from build123d import *

# Parameters (mm, degrees)
CYLINDER_R        = 0.4
CYLINDER_DEPTH    = 4.6
CYLINDER001_R     = 0.4
CYLINDER001_DEPTH = 4.6
CYLINDER002_R     = 0.4
CYLINDER002_DEPTH = 4.6
CYLINDER003_R     = 0.4
CYLINDER003_DEPTH = 4.6
BOX003_W          = 12.8
BOX003_H          = 16.299999
BOX003_DEPTH      = 2
BOX002_W          = 3.4
BOX002_H          = 18.299999
BOX002_DEPTH      = 2
BOX001_W          = 3.4
BOX001_H          = 18.299999
BOX001_DEPTH      = 2
BOX_W             = 12.8
BOX_H             = 18.299999
BOX_DEPTH         = 20.299999
CHAMFER_SIZE      = 3
FILLET_R          = 0.6


with BuildPart() as pin4:
    # Cylinder → Cylinder (new body)
    with BuildSketch(Plane(origin=(1.4, 1.65, -2.6), x_dir=(1, 0, 0), z_dir=(0, 0, 1))):
        Circle(CYLINDER_R)
    extrude(amount=CYLINDER_DEPTH)


with BuildPart() as pin3:
    # Cylinder001 → Cylinder001 (new body)
    with BuildSketch(Plane(origin=(11.4, 1.65, -2.6), x_dir=(1, 0, 0), z_dir=(0, 0, 1))):
        Circle(CYLINDER001_R)
    extrude(amount=CYLINDER001_DEPTH)


with BuildPart() as pin2:
    # Cylinder002 → Cylinder002 (new body)
    with BuildSketch(Plane(origin=(11.4, 16.65, -2.6), x_dir=(1, 0, 0), z_dir=(0, 0, 1))):
        Circle(CYLINDER002_R)
    extrude(amount=CYLINDER002_DEPTH)


with BuildPart() as pin1:
    # Cylinder003 → Cylinder003 (new body)
    with BuildSketch(Plane(origin=(1.4, 16.65, -2.6), x_dir=(1, 0, 0), z_dir=(0, 0, 1))):
        Circle(CYLINDER003_R)
    extrude(amount=CYLINDER003_DEPTH)


with BuildPart() as box003:
    # Box003 → Box003 (new body)
    with BuildSketch(Plane(origin=(0, 1, 0), x_dir=(1, 0, 0), z_dir=(0, 0, 1))):
        with Locations((6.4, 8.149999)):
            Rectangle(BOX003_W, BOX003_H)
    extrude(amount=BOX003_DEPTH)


with BuildPart() as right_cutout:
    # Box002 → Box002 (new body)
    with BuildSketch(Plane(origin=(9.4, 0, 0), x_dir=(1, 0, 0), z_dir=(0, 0, 1))):
        with Locations((1.7, 9.149999)):
            Rectangle(BOX002_W, BOX002_H)
    extrude(amount=BOX002_DEPTH)


with BuildPart() as left_cutout:
    # Box001 → Box001 (new body)
    with BuildSketch(Plane.XY):
        with Locations((1.7, 9.149999)):
            Rectangle(BOX001_W, BOX001_H)
    extrude(amount=BOX001_DEPTH)


with BuildPart() as obj1:
    # Box → Box (new body)
    with BuildSketch(Plane.XY):
        with Locations((6.4, 9.149999)):
            Rectangle(BOX_W, BOX_H)
    extrude(amount=BOX_DEPTH)

    # Cut: cut left_cutout
    add(left_cutout.part, mode=Mode.SUBTRACT)

    # Cut001: cut right_cutout
    add(right_cutout.part, mode=Mode.SUBTRACT)

    # Cut002: cut Box003
    add(box003.part, mode=Mode.SUBTRACT)

    # Chamfer
    chamfer_edges = [obj1.edges().sort_by_distance(p)[0] for p in [
        (6.4, 18.299999, 20.299999),
    ]]
    chamfer(chamfer_edges, length=CHAMFER_SIZE)

    # Fillet
    fillet_edges = [obj1.edges().sort_by_distance(p)[0] for p in [
        (0, 7.65, 20.299999),
        (6.4, 0, 20.299999),
        (12.8, 7.65, 20.299999),
        (0, 0, 11.15),
        (0, 18.299999, 9.65),
        (12.8, 0, 11.15),
        (12.8, 18.299999, 9.65),
    ]]
    fillet(fillet_edges, radius=FILLET_R)

    # Fusion: union Pin4, Pin3, Pin2, Pin1
    add(pin4.part)
    add(pin3.part)
    add(pin2.part)
    add(pin1.part)


solid = obj1.part
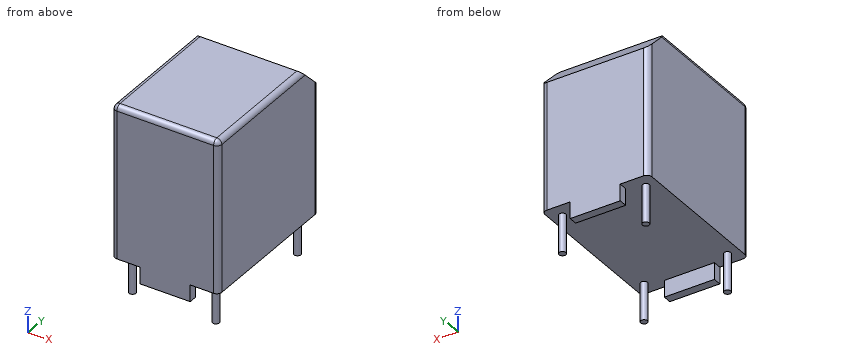
Work out the finished part from the listing and answer in its coordinate system (mm). Give positions to 0.01 mm unless a question says otherwise; leave off trailing zeros. Loops run counter-clockwise (first coordinate to the right, second up) from the corner with the lowest first, then second, coordinate; pieces in that order, holes last. Notation, with made-up numbers: (78.5, -26.75) -> (131.5, -26.75) arc R10 cw to (131.5, -17.75) -> close; hole circle Ø8 at (60.25, 5). An arc over 180 degrees is marked (long way). Use a Markdown table: item, result. Add a question column.
1. Find the intervals of material crossed by probe 1 along Z at (x, y) = (3.5, 14.5); probe 2 along Y at (x, z) = (8.75, 0.5); probe 3 along Y at (x, z) = (12.25, 9.25), in increasing order.
2. Flat-ended cylindrical pins translate along their axes: pin 1 Ø5 at (x, y) = (10, 3.5) entering from -Z; pin 2 Ø0.5 at (x, y) = (5.5, 0.5) entering from -Z; pin 3 Ø1.1 at (y, z) = (0.5, 1) entering from -X; pin 4 Ø1.5 at (x, y) = (7.5, 8.5) entering from -Z. Find the tip coordinate at first contact, or state that the pin passes through.
3. Section D-D on z = 18.5 is taken. Determine the outline of the cut face in (x, y), and give its area (3 significant figures).
4. Section A-A on z = 1 is taken. Determine the outline of the cut face in (x, y).
5. Section B-B on x = 4.75 is taken. Determine the outline of the cut face in (y, z).
6. Section C-C on y = 1.65 is taken. Determine the outline of the cut face in (x, z), and give its area (3 significant figures).
Results below:
| question | item | result |
|---|---|---|
| 1 | probe 1 | z = 2 to 20.3 |
| 1 | probe 2 | y = 0 to 1, 17.3 to 18.3 |
| 1 | probe 3 | y = 0 to 18.3 |
| 2 | pin 1 | stops at z = -2.6 |
| 2 | pin 2 | stops at z = 0 |
| 2 | pin 3 | stops at x = 3.4 |
| 2 | pin 4 | stops at z = 2 |
| 3 | outline | (0, 0.6) arc R0.6 ccw to (0.6, 0) -> (12.2, 0) arc R0.6 ccw to (12.8, 0.6) -> (12.8, 17.1) -> (0, 17.1) -> close |
| 3 | area | 219 mm^2 |
| 4 | outline | circle Ø0.8 at (1.4, 1.65); circle Ø0.8 at (1.4, 16.65); (3.4, 0) -> (9.4, 0) -> (9.4, 1) -> (3.4, 1) -> close; (3.4, 17.3) -> (9.4, 17.3) -> (9.4, 18.3) -> (3.4, 18.3) -> close; circle Ø0.8 at (11.4, 1.65); circle Ø0.8 at (11.4, 16.65) |
| 5 | outline | (0, 0) -> (1, 0) -> (1, 2) -> (17.3, 2) -> (17.3, 0) -> (18.3, 0) -> (18.3, 17.3) -> (15.3, 20.3) -> (0.6, 20.3) arc R0.6 ccw to (0, 19.7) -> close |
| 6 | outline | (0, 2) -> (1, 2) -> (1, -2.6) -> (1.8, -2.6) -> (1.8, 2) -> (11, 2) -> (11, -2.6) -> (11.8, -2.6) -> (11.8, 2) -> (12.8, 2) -> (12.8, 19.7) arc R0.6 ccw to (12.2, 20.3) -> (0.6, 20.3) arc R0.6 ccw to (0, 19.7) -> close |
| 6 | area | 241 mm^2 |
